Input: dimensioned drawing with shaded views. Units: mm. Origin: part minimum x, y, z. Round coordinates to 2 decimals unless told otherwise and drop trailing zeros. Write each loop counter-clockwise with the first axis right and the second up, starting at its lowest first coordinate (ties: lowest second). Pieces come first, ordered by that corner, then holes. Notation, with made-up numbers: (4, 35.5) -> (19, 35.5) arc R26 cw to (19, 69.5) -> close; hole circle Ø11 at (40.5, 20). An arc over 180 degrees is marked (long way). One line per item, written item: value. Start each with the question number.
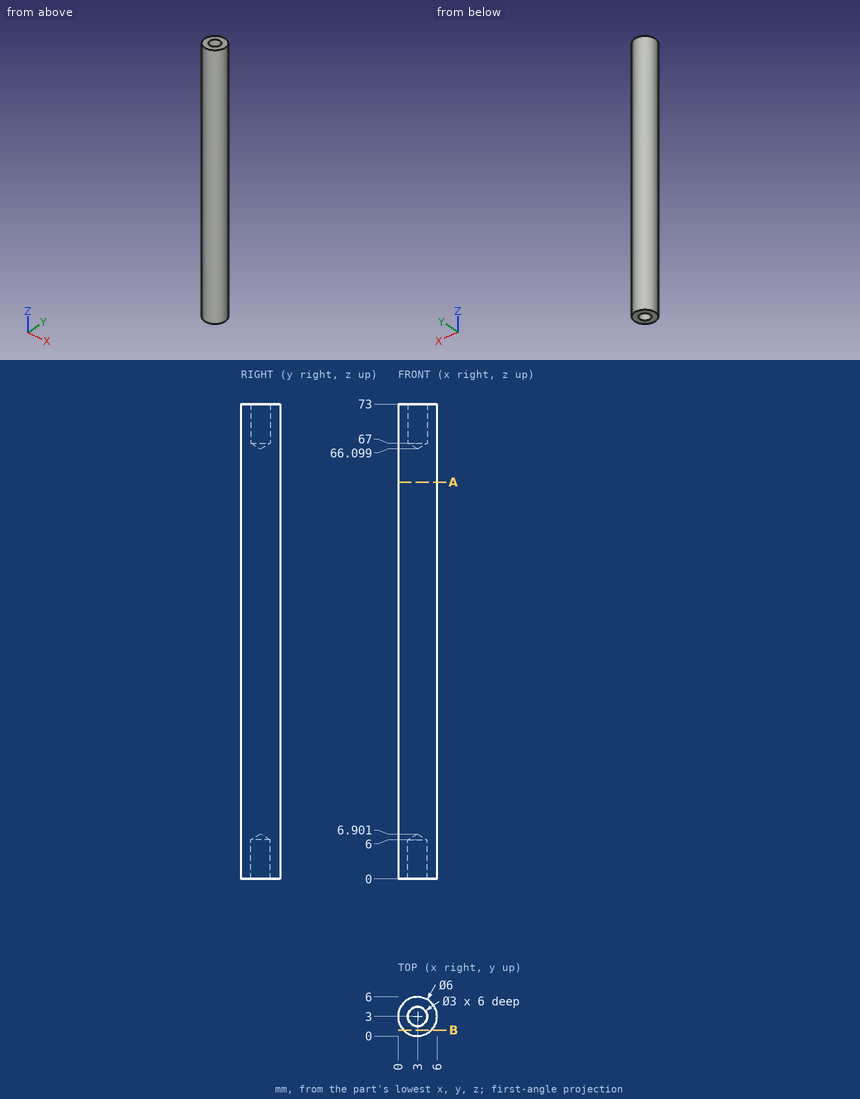
(1) Line query: probe 1 along Y at (x, z) = (3, 68.8); probe 2 along Y at (x, z) = (0.4, 53) (1 decimal). Output: solid intervals per line, ascending.
(2) Section query B-B (y = 0.9). Output: boundary loops of the cut face in (x, z), and give its area (3 significant figures).
(3) Section query A-A (z = 61). Output: boundary loops of the cut face in (x, y).
(4) Pin query (flat end, axial travel): pin 1 (2 mm diameter, centred on x = 4.5, z = 58.5, fed in from -Y); pin 2 (2 mm diameter, centred on x = 5, z = 64.5, fed in from +Y); pin 3 (2.5 mm diameter, centred on x = 3, y = 3, fed in from -Z). Return the tip coordinate at first contact, or that it passes through.
Results list:
1. probe 1: y = 0 to 1.5, 4.5 to 6
1. probe 2: y = 1.5 to 4.5
2. outline: (0.86, 0) -> (5.14, 0) -> (5.14, 73) -> (0.86, 73) -> close
2. area: 313 mm^2
3. outline: circle Ø6 at (3, 3)
4. pin 1: stops at y = 0.04
4. pin 2: stops at y = 5.83
4. pin 3: stops at z = 6.15
